Verification items for the finished model (mm, model axes). Face numbers are marked on the shaded views. A direction names the side the tool comes from. Give positions to 0.01 mm unless a question says otherwise; leave off trailing zeros. Order: outer loops, then holes, each group sorted by start corner. A loop starts at its lowest first (then second) coordinate and runs counter-clockwise, first axis right, second up. Notation, with made-up numbers: M 81,-38.75 L 120,-38.75 A14 cw 120,-17.75 Z; hole C 3.25,13 d9. An arc over 180 degrees is marked long. Answer as a JSON object with one key per item and string values.
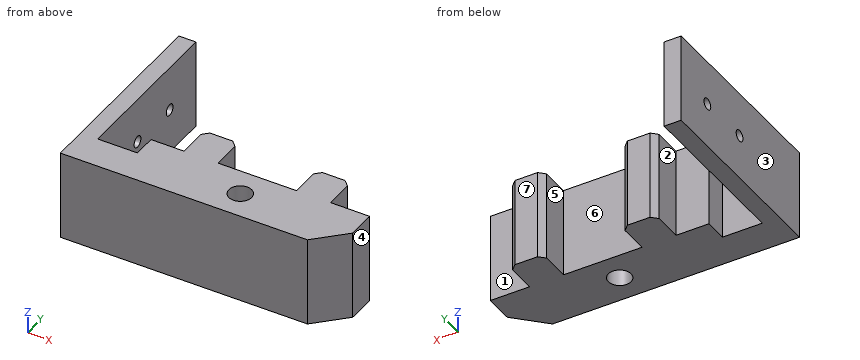
```python
from build123d import *

# Parameters (mm, degrees)
F1_DEPTH  = 15.75
F4_D      = 4
F5_DEPTH  = 3
F6_W      = 3
F6_H      = 15.75
F7_DEPTH  = 25
F9_D      = 2
F10_W     = 6
F10_H     = 4
F11_DEPTH = 15.751
F12_SIZE  = 1
F13_SIZE  = 5
F14_DEPTH = 1
F15_DEPTH = 1


with BuildPart() as f1:
    # F0 (on Top) → F1 (new body)
    with BuildSketch(Plane.XY):
        Polygon((0, 0), (44.5, 0), (44.5, 10), (37.6, 10), (37.6, 16), (31.6, 16), (31.6, 10), (17.8, 10), (17.8, 16), (11.8, 16), (11.8, 10), (0, 10), align=None)
    extrude(amount=F1_DEPTH)

    # F4 (through all)
    with Locations(Plane.XY.offset(15.75)):
        with Locations((24.7, 5)):
            Hole(F4_D / 2)

    # F5 (add): a face of the model
    f5_faces = [f1.faces().sort_by_distance(p)[0] for p in [
        (0, 5, 7.875),
    ]]
    extrude(f5_faces, amount=F5_DEPTH)

    # F6 (on face) → F7 (join)
    with BuildSketch(Plane(origin=(0, 10, 0), x_dir=(-1, 0, 0), z_dir=(0, 1, 0))):
        with Locations((1.5, 7.875)):
            Rectangle(F6_W, F6_H)
    extrude(amount=F7_DEPTH)

    # F9 (through all)
    with Locations(Plane.YZ):
        with Locations((27.25, 7.875), (17.75, 7.875)):
            Hole(F9_D / 2)

    # F10 (on face) → F11 (cut, through all)
    with BuildSketch(Plane.XY.offset(15.75)):
        with Locations((3, 8)):
            Rectangle(F10_W, F10_H)
    extrude(amount=-F11_DEPTH, mode=Mode.SUBTRACT)

    # F12
    f12_edges = [f1.edges().sort_by_distance(p)[0] for p in [
        (11.8, 16, 7.875),
        (17.8, 16, 7.875),
        (31.6, 16, 7.875),
        (37.6, 16, 7.875),
    ]]
    chamfer(f12_edges, length=F12_SIZE)

    # F13
    f13_edges = [f1.edges().sort_by_distance(p)[0] for p in [
        (44.5, 0, 7.875),
    ]]
    chamfer(f13_edges, length=F13_SIZE)

    # F14 (add): a face of the model
    f14_faces = [f1.faces().sort_by_distance(p)[0] for p in [
        (-3, 0.3838049635, 7.875),
    ]]
    extrude(f14_faces, amount=F14_DEPTH)

    # F15 (cut): a face of the model
    f15_faces = [f1.faces().sort_by_distance(p)[0] for p in [
        (0, 20.4721036707, 7.875),
    ]]
    extrude(f15_faces, amount=-F15_DEPTH, mode=Mode.SUBTRACT)


solid = f1.part
```
Q1. Release check for a two-part mould opening along X. For the marked faces 4, 5, 6 and 7 record: +X half, -X half, draft (parallel to the pull), parting line (faces both ways), or undercut.
Resolved:
{"face 4": "+X half", "face 5": "undercut", "face 6": "undercut", "face 7": "draft"}
Q2. Section check C-C on z = 6. Record the cut outline in (x, y).
Resolved:
{"outline": "M -4,0 L 39.5,0 L 44.5,5 L 44.5,10 L 37.6,10 L 37.6,15 L 36.6,16 L 32.6,16 L 31.6,15 L 31.6,10 L 17.8,10 L 17.8,15 L 16.8,16 L 12.8,16 L 11.8,15 L 11.8,10 L 6,10 L 6,6 L -1,6 L -1,35 L -4,35 Z; hole C 24.7,5 d4"}
Q3. Section check A-A on x = 24.7. Record the cut outline in (y, z), then the cut area to 3 significant figures.
Resolved:
{"outline": "M 0,0 L 3,0 L 3,15.75 L 0,15.75 Z; M 7,0 L 10,0 L 10,15.75 L 7,15.75 Z", "area": "94.5 mm²"}
Q4. Tool access check on the marked faces 1, 2 and 3. Record the directions out of +Z, -Z, +X, -X, +Y, -Y that give a thin tool (end or side, any length) a straight path to the whole face; none if there is none.
Resolved:
{"face 1": "+Z, -Z, +X, +Y", "face 2": "+Z, -Z, +Y", "face 3": "+Z, -Z, -X, +Y, -Y"}
Q5. Gauge pin test, flat ends, axial feed: pin 1 Ø2.5 at (y, z) = (27.25, 7.875) entering from +X; pin 2 Ø5.5 at (y, z) = (13, 5.5) entering from +X; pin 3 Ø6 at (x, z) = (38, 13.5) entering from +Y. Record the tip position at first contact, or that the pin passes through.
Resolved:
{"pin 1": "stops at x = -1", "pin 2": "stops at x = 37.6", "pin 3": "stops at y = 16"}
Q6. Material ranges on L1, parallel to X at y = 14, z = 1.25; L2, parallel to Z at x = -1.85, y = 17.75 (3 decimals); L3, parallel to Y at x = 29.5, z = 6.75, recorded low to high.
Resolved:
{"L1": "x = -4 to -1, 11.8 to 17.8, 31.6 to 37.6", "L2": "z = 0 to 6.875, 8.875 to 15.75", "L3": "y = 0 to 10"}
Q7. Section check B-B on y = 27.25. Record the cut outline in (x, z) (3 decimals).
Resolved:
{"outline": "M -4,0 L -1,0 L -1,6.875 L -4,6.875 Z; M -4,8.875 L -1,8.875 L -1,15.75 L -4,15.75 Z"}
Q8. Section check D-D on y = 10.5. Record the cut outline in (x, z), then the cut area to 3 significant figures.
Resolved:
{"outline": "M -4,0 L -1,0 L -1,15.75 L -4,15.75 Z; M 11.8,0 L 17.8,0 L 17.8,15.75 L 11.8,15.75 Z; M 31.6,0 L 37.6,0 L 37.6,15.75 L 31.6,15.75 Z", "area": "236 mm²"}
